Verification items for this drawing (mm, ordinates from the low corner). Give positions to 0.01 mm unless a question says otherwise; leave off trailing zeros. Order: outer loops, then holes, each group sorted by start corner. A loop starts at its lowest first (then second) coordinate and runs counter-clockwise, first axis right, second up.
(1) Scan lines: L1, parallel to X at y = 4, z = 92 (1 decimal); L2, parallel to Z at x = 119, y = 22 (1 decimal); L3, parallel to Z at x = 102, y = 7.25 (1 decimal). Record each from-to range of solid material in increasing order.
(2) Gauge pin test, flat ends, axial feed: pin 1 (12 mm diameter, centred on x = 123, y = 10, fed in from -Z); pin 2 (1 mm diameter, centred on y = 8.5, z = 101.5, fed in from +X); pin 3 (5 mm diameter, centred on x = 40, z = 113, fed in from -Y); pin 4 (2 mm diameter, centred on x = 118.5, z = 69, fed in from +Y). Record the tip position at first contact, or that the pin passes through.
(3) Sectioned sample at A-A on y = 14.75. Record the cut outline in (x, z) (1 decimal).
(4) Mould release check, pull along X, two halves, no side actions. Record for the marked faces 1, 2, 3 and 4: pulls with the +X half, pulls with the -X half, needs draft (parallel to the pull), parting line crosses it, or undercut.
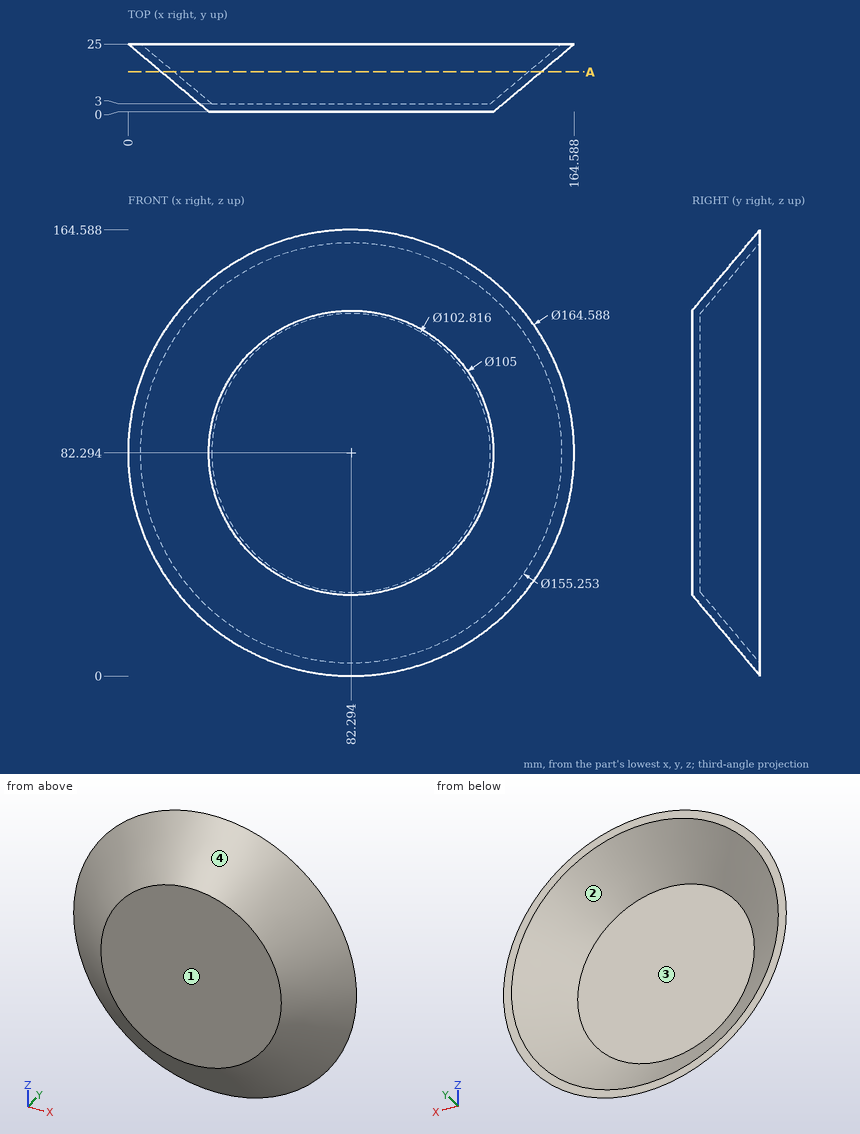
Ans:
1. L1: x = 25.9 to 30.6, 134 to 138.7
1. L2: z = 12.7 to 18, 146.6 to 151.9
1. L3: z = 24.4 to 29.4, 135.2 to 140.2
2. pin 1: stops at z = 22.55
2. pin 2: stops at x = 142.55
2. pin 3: stops at y = 0
2. pin 4: stops at y = 3
3. outline: circle Ø140.2 at (82.3, 82.3); hole circle Ø130.8 at (82.3, 82.3)
4. face 1: needs draft
4. face 2: undercut
4. face 3: undercut
4. face 4: parting line crosses it
